Here's how the part is built. I have some questions about the finished solid (model axes, mm). A direction names the side the tool comes from. Round coordinates to 2 decimals unless told otherwise and drop trailing zeros. Loops run counter-clockwise (first coordinate to the right, second up) from the corner with the lowest first, then second, coordinate; pieces in that order, holes last. Notation, with made-up numbers: M 48.5,54 L 102.5,54 A35 cw 102.5,87 Z; hole C 48.25,12.25 d2. An arc over 180 degrees is marked long. Use a Markdown table: item, result.
```python
from build123d import *

# Parameters (mm, degrees)
SKETCH1_W           = 120
SKETCH1_H           = 75
SKETCH1_R           = 3
BOSS_EXTRUDE1_DEPTH = 10
SKETCH2_R           = 2.5
CUT_EXTRUDE1_DEPTH  = 10
SKETCH3_R           = 1.5
CUT_EXTRUDE2_DEPTH  = 10
LPATTERN1_COUNT     = 2
LPATTERN1_PITCH     = 110
SKETCH4_W           = 120
SKETCH4_H           = 130
BOSS_EXTRUDE2_DEPTH = 10
SKETCH5_R           = 1.5
CUT_EXTRUDE3_DEPTH  = 10
LPATTERN2_COUNT     = 2
LPATTERN2_PITCH     = 110
SKETCH6_R           = 2.5
CUT_EXTRUDE4_DEPTH  = 10
SKETCH7_R           = 1.5
CUT_EXTRUDE5_DEPTH  = 10


with BuildPart() as part:
    # Sketch1 → Boss-Extrude1 (new body)
    with BuildSketch(Plane.XY):
        Rectangle(SKETCH1_W, SKETCH1_H)
        with Locations((-44, 31.5)):
            Circle(SKETCH1_R, mode=Mode.SUBTRACT)
        with Locations((44, 31.5)):
            Circle(SKETCH1_R, mode=Mode.SUBTRACT)
        with Locations((-44, -31.5)):
            Circle(SKETCH1_R, mode=Mode.SUBTRACT)
        with Locations((44, -31.5)):
            Circle(SKETCH1_R, mode=Mode.SUBTRACT)
    extrude(amount=BOSS_EXTRUDE1_DEPTH)

    # Sketch2 → Cut-Extrude1 (cut)
    with BuildSketch(Plane.XY.offset(10)):
        with Locations((0, 10)):
            Circle(SKETCH2_R)
        with Locations((0, -10)):
            Circle(SKETCH2_R)
    extrude(amount=-CUT_EXTRUDE1_DEPTH, mode=Mode.SUBTRACT)

    # Sketch3 → Cut-Extrude2 (cut)
    with BuildSketch(Plane(origin=(60, 0, 0), x_dir=(0, 0, -1), z_dir=(1, 0, 0))):
        with Locations(Location((-5, 17.5, 0), (0, 0, 90))):
            Circle(SKETCH3_R)
        with Locations(Location((-5, -17.5, 0), (0, 0, 90))):
            Circle(SKETCH3_R)
    cut_extrude2 = extrude(amount=-CUT_EXTRUDE2_DEPTH, mode=Mode.SUBTRACT)

    # LPattern1: Cut-Extrude2 ×2
    with Locations(*[(-i * LPATTERN1_PITCH, 0, 0) for i in range(1, LPATTERN1_COUNT)]):
        add(cut_extrude2, mode=Mode.SUBTRACT)

    # Sketch4 → Boss-Extrude2 (add)
    with BuildSketch(Plane(origin=(0, 37.5, 0), x_dir=(1, 0, 0), z_dir=(0, 1, 0))):
        with Locations((0, -50)):
            Rectangle(SKETCH4_W, SKETCH4_H)
    extrude(amount=BOSS_EXTRUDE2_DEPTH)

    # Sketch5 → Cut-Extrude3 (cut)
    with BuildSketch(Plane(origin=(60, 0, 0), x_dir=(0, 0, -1), z_dir=(1, 0, 0))):
        with Locations(Location((-105, 42.5, 0), (0, 0, 90))):
            Circle(SKETCH5_R)
        with Locations(Location((-25, 42.5, 0), (0, 0, 90))):
            Circle(SKETCH5_R)
    cut_extrude3 = extrude(amount=-CUT_EXTRUDE3_DEPTH, mode=Mode.SUBTRACT)

    # LPattern2: Cut-Extrude3 ×2
    with Locations(*[(-i * LPATTERN2_PITCH, 0, 0) for i in range(1, LPATTERN2_COUNT)]):
        add(cut_extrude3, mode=Mode.SUBTRACT)

    # Sketch6 → Cut-Extrude4 (cut)
    with BuildSketch(Plane(origin=(0, 47.5, 0), x_dir=(1, 0, 0), z_dir=(0, 1, 0))):
        with Locations(Location((-25, -98, 0), (0, 0, 270))):
            Circle(SKETCH6_R)
        with Locations(Location((25, -98, 0), (0, 0, 270))):
            Circle(SKETCH6_R)
        with Locations(Location((-25, -58, 0), (0, 0, 270))):
            Circle(SKETCH6_R)
        with Locations(Location((25, -58, 0), (0, 0, 270))):
            Circle(SKETCH6_R)
    extrude(amount=-CUT_EXTRUDE4_DEPTH, mode=Mode.SUBTRACT)

    # Sketch7 → Cut-Extrude5 (cut)
    with BuildSketch(Plane(origin=(0, 47.5, 0), x_dir=(1, 0, 0), z_dir=(0, 1, 0))):
        with Locations(Location((-5, 9, 0), (0, 0, 270))):
            Circle(SKETCH7_R)
        with Locations(Location((5, 9, 0), (0, 0, 270))):
            Circle(SKETCH7_R)
    extrude(amount=-CUT_EXTRUDE5_DEPTH, mode=Mode.SUBTRACT)


solid = part.part
```
Q1. Imagine slicing it at B-B, the plane x = 25. Please give me the cut outline in (y, z), then the cut area to 3 significant figures.
Return value:
| item | result |
|---|---|
| outline | M -37.5,0 L 37.5,0 L 37.5,-15 L 47.5,-15 L 47.5,55.5 L 37.5,55.5 L 37.5,10 L -37.5,10 Z; M 37.5,60.5 L 47.5,60.5 L 47.5,95.5 L 37.5,95.5 Z; M 37.5,100.5 L 47.5,100.5 L 47.5,115 L 37.5,115 Z |
| area | 1,950 mm^2 |
Q2. Imagine slicing it at A-A, the plane y = 10. Please give me the cut outline in (x, z).
Return value:
| item | result |
|---|---|
| outline | M -60,0 L -2.5,0 L -2.5,10 L -60,10 Z; M 2.5,0 L 60,0 L 60,10 L 2.5,10 Z |
Q3. Imagine slicing it at D-D, the plane x = -35. Please give me the cut outline in (y, z).
Return value:
| item | result |
|---|---|
| outline | M -37.5,0 L 37.5,0 L 37.5,-15 L 47.5,-15 L 47.5,115 L 37.5,115 L 37.5,10 L -37.5,10 Z |
Q4. Will these pins go through, and if not, where does the flat tip stop? P1, Ø5, axis at x = 5, z = -9, coming from the -Y side; P2, Ø4.5, axis at x = 0, y = 10, coming from the +Z side; P3, Ø1.5, axis at y = 17.5, z = 5, coming from the -X side; P4, Ø22.5, axis at x = 28.5, y = -3.5, coming from the -Z side.
Return value:
| item | result |
|---|---|
| P1 | stops at y = 37.5 |
| P2 | passes through |
| P3 | stops at x = -50 |
| P4 | stops at z = 0 |
Q5. For faces 1 (the flat face through (50, 42, 105)), 2 (the cylindrical face through (-22.52, 42.57, 97.67)), 3 (the cylindrical face through (-54.93, 42.305, 106.487)), which set-ups out of +Z, -Z, +X, -X, +Y, -Y let a thin tool reach every point of the face, with its end or its side?
Return value:
| item | result |
|---|---|
| face 1 | +X |
| face 2 | +Y, -Y |
| face 3 | -X |
Q6. We'd pull the mould along Y, two halves only. Please class faces 4 (the flat face through (-50, 17, 5)), 5 (the flat face through (-1, 1, 10)), 6 (the flat face through (-1, 47.5, 49)): pulls with the +Y half, pulls with the -Y half, needs draft (parallel to the pull), parting line crosses it, or undercut.
Return value:
| item | result |
|---|---|
| face 4 | undercut |
| face 5 | needs draft |
| face 6 | pulls with the +Y half |
Q7. Imagine slicing it at C-C, the plane z = 98. Please give me the cut outline in (x, y), then the cut area to 3 significant figures.
Return value:
| item | result |
|---|---|
| outline | M -60,37.5 L -27.5,37.5 L -27.5,47.5 L -60,47.5 Z; M -22.5,37.5 L 22.5,37.5 L 22.5,47.5 L -22.5,47.5 Z; M 27.5,37.5 L 60,37.5 L 60,47.5 L 27.5,47.5 Z |
| area | 1,100 mm^2 |
Q8. I need wall thicknesses on line 1 (X direction, y = 44, z = -9); line 2 (Y direction, x = -44, z = 7.5); line 3 (X direction, y = 44.75, z = 58). Which ranges of each line are inside material? Lowest first, please. Write a range as from..to.
Return value:
| item | result |
|---|---|
| line 1 | x = -60..-6.5, -3.5..3.5, 6.5..60 |
| line 2 | y = -37.5..-34.5, -28.5..28.5, 34.5..47.5 |
| line 3 | x = -60..-27.5, -22.5..22.5, 27.5..60 |
